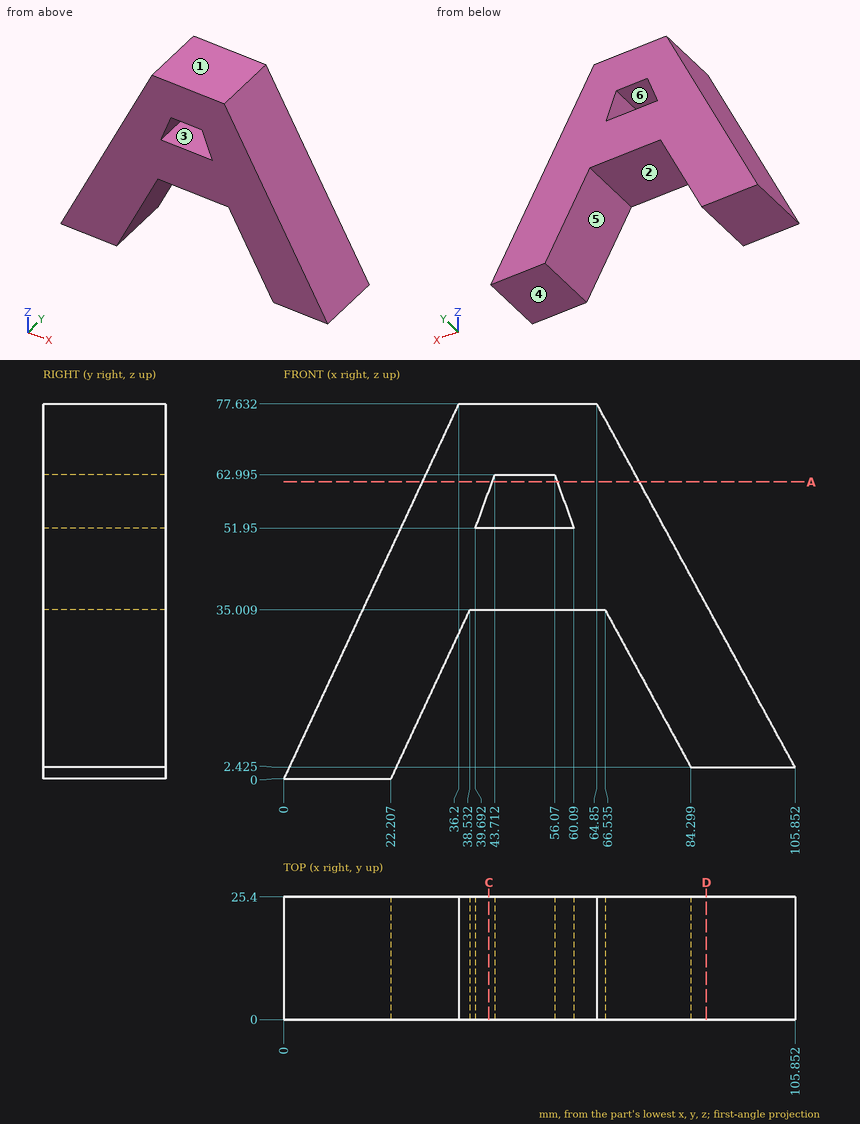
Job drawing, mm, ordinate dimensions from the low corner. One solid piece. A direction names the side the tool comes from. Coordinates: 2 decimals unless noted, no trailing zeros. Write each loop counter-clockwise with the first axis right and the second up, starting at its lowest first coordinate (ties: lowest second). Pieces come first, ordered by that corner, then holes. Notation, with made-up numbers: (-16.75, 77.5) - (-9.75, 77.5) arc R32 cw to (-9.75, 113.5) - close; hole circle Ø11 at (66.5, 84). An arc over 180 degrees is marked (long way). Use a Markdown table: item, result. Add a question column.
Item 1: Flat gauge pins, fed straight in: pin 1 (5 mm diameter, centred on y = 4, z = 39, fed in from -X); pin 2 (12.5 mm diameter, centred on x = 47.5, y = 7, fed in from -Z); pin 3 (6.5 mm diameter, centred on x = 96.5, y = 10.5, fed in from -Z) (1 decimal). Where does each tip first touch, or does it go through?
Item 2: Band-saw the part on D-D, the plane x = 87.5. Give the cut face in (y, z) (1 decimal), and give its area (3 significant figures).
Item 3: Band-saw the part on C-C, the plane x = 42.5. Give the cut face in (y, z).
Item 4: Mould opens along Z. For the marked faces 1, 2 and 3 say: pulls with the +Z half, pulls with the -Z half, needs draft (parallel to the pull), parting line crosses it, or undercut.
Item 5: 3-axis set-ups, long thin cutter, end or side, ignore diameter. For the marked faces 4, 5 and 6: which of +Z, -Z, +X, -X, +Y, -Y reach the whole face in a straight line?
Item 6: Drill centre lines: L1, parallel to X at y = 12.75, z = 14.5 (1 decimal); L2, parallel to X at y = 23, z = 58 (1 decimal); L3, parallel to X at y = 22.5, z = 42 (1 decimal). Where is each one in solid material? Low to high. Write a range as from..to.
Item 7: Band-saw the part on A-A, the plane z = 61.5. Give the cut face in (x, y) (1 decimal).
Numbers:
| question | item | result |
|---|---|---|
| 1 | pin 1 | x = 17.02 |
| 1 | pin 2 | z = 35.01 |
| 1 | pin 3 | z = 2.4 |
| 2 | outline | (0, 2.4) - (25.4, 2.4) - (25.4, 36.1) - (0, 36.1) - close |
| 2 | area | 855 mm2 |
| 3 | outline | (0, 35.01) - (25.4, 35.01) - (25.4, 51.95) - (0, 51.95) - close; (0, 59.67) - (25.4, 59.67) - (25.4, 77.63) - (0, 77.63) - close |
| 4 | face 1 | pulls with the +Z half |
| 4 | face 2 | pulls with the -Z half |
| 4 | face 3 | undercut |
| 5 | face 4 | -Z, +X, +Y, -Y |
| 5 | face 5 | -Z, +Y, -Y |
| 5 | face 6 | +Y, -Y |
| 6 | L1 | 6.8..29, 77.7..99.3 |
| 6 | L2 | 27..41.9, 57.9..75.6 |
| 6 | L3 | 19.6..84.3 |
| 7 | outline | (28.7, 0) - (43.2, 0) - (43.2, 25.4) - (28.7, 25.4) - close; (56.6, 0) - (73.6, 0) - (73.6, 25.4) - (56.6, 25.4) - close |
